Geometry check sheet. Reference: the model listing, model coordinates, mm. Face numbers are marked on the shaded views. Give positions to 0.01 mm unless a question says otherwise; leave off trailing zeros. Loops run counter-clockwise (first coordinate to the right, second up) from the corner with the lowest first, then second, coordinate; pieces in that order, holes last.
1. Go/stop test with flat-tipped pins: pin 1 Ø3 at (y, z) = (4, 6) entering from -X; pin 2 Ø2 at (x, y) = (-1, 2) entering from +Z; pin 3 Ø1 at (y, z) = (1, 1.5) entering from +X. Record where each tip stops, or that it passes through.
2. Cross-section at A-A, the plane x = 0. Record the cut outline in (y, z).
3. Cross-section at B-B, the plane z = 0. Record the cut outline in (x, y).
4. Material ranges on L1, parallel to X at y = 3.5, z = 0; L2, parallel to Z at x = 0, y = 2.25; L3, parallel to Y at x = 7.75, z = -6.25, recorded low to high.
5. Cross-section at C-C, the plane y = 3.8. Record the cut outline in (x, z), plus the area to 3 significant figures.
6. Release check for a two-part mould opening along X. For the marked faces 1, 2 and 3 record: +X half, -X half, draft (parallel to the pull), parting line (faces both ways), or undercut.
from build123d import *


with BuildPart() as part:
    # Sketch1 → Revolve1 (revolve)
    with BuildSketch(Plane.XY):
        with BuildLine():
            Line((6, 0.2), (6, 4.8))
            ThreePointArc((6, 4.8), (6.058578644, 4.941421356), (6.2, 5))
            Line((6.2, 5), (10.3, 5))
            ThreePointArc((10.3, 5), (10.441421356, 4.941421356), (10.5, 4.8))
            Line((10.5, 4.8), (10.5, 3))
            Line((10.5, 3), (9.411915576, 3))
            Line((9.411915576, 3), (9.411915576, 2))
            Line((9.411915576, 2), (10.5, 2))
            Line((10.5, 2), (10.5, 0.2))
            ThreePointArc((10.5, 0.2), (10.441421356, 0.058578644), (10.3, 0))
            Line((10.3, 0), (6.2, 0))
            ThreePointArc((6.2, 0), (6.058578644, 0.058578644), (6, 0.2))
        make_face()
    revolve(axis=Axis((0, 0, 0), (0, 1, 0)))


solid = part.part
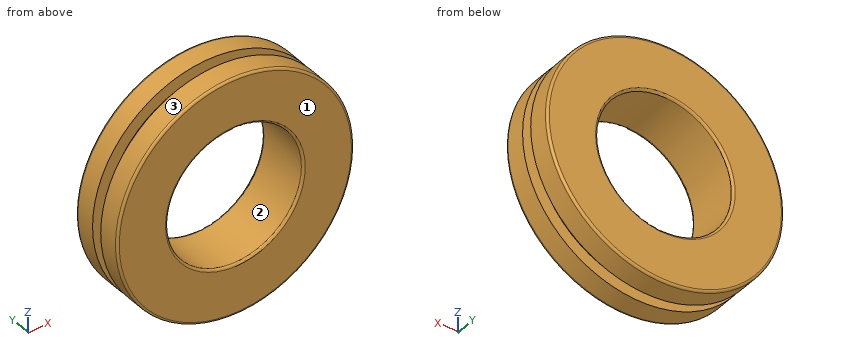
Result:
1. pin 1: stops at x = -9.49
1. pin 2: stops at z = 10.5
1. pin 3: stops at x = 10.45
2. outline: (0, -10.3) arc R0.2 ccw to (0.2, -10.5) - (2, -10.5) - (2, -9.41) - (3, -9.41) - (3, -10.5) - (4.8, -10.5) arc R0.2 ccw to (5, -10.3) - (5, -6.2) arc R0.2 ccw to (4.8, -6) - (0.2, -6) arc R0.2 ccw to (0, -6.2) - close; (0, 6.2) arc R0.2 ccw to (0.2, 6) - (4.8, 6) arc R0.2 ccw to (5, 6.2) - (5, 10.3) arc R0.2 ccw to (4.8, 10.5) - (3, 10.5) - (3, 9.41) - (2, 9.41) - (2, 10.5) - (0.2, 10.5) arc R0.2 ccw to (0, 10.3) - close
3. outline: (-10.5, 0.2) arc R0.2 ccw to (-10.3, 0) - (-6.2, 0) arc R0.2 ccw to (-6, 0.2) - (-6, 4.8) arc R0.2 ccw to (-6.2, 5) - (-10.3, 5) arc R0.2 ccw to (-10.5, 4.8) - (-10.5, 3) - (-9.41, 3) - (-9.41, 2) - (-10.5, 2) - close; (6, 0.2) arc R0.2 ccw to (6.2, 0) - (10.3, 0) arc R0.2 ccw to (10.5, 0.2) - (10.5, 2) - (9.41, 2) - (9.41, 3) - (10.5, 3) - (10.5, 4.8) arc R0.2 ccw to (10.3, 5) - (6.2, 5) arc R0.2 ccw to (6, 4.8) - close
4. L1: x = -10.5 to -6, 6 to 10.5
4. L2: z = -9.41 to -6, 6 to 9.41
4. L3: y = 0 to 2, 3 to 5
5. outline: circle Ø21 at (0, 0); hole circle Ø12 at (0, 0)
5. area: 233 mm2
6. face 1: draft
6. face 2: undercut
6. face 3: parting line
